Geometry check sheet. Reference: drawing and pictorial views, mm from the part's lowest x, y, z. A direction names the side the tool comes from. Coordinates: 2 decimals unless noted, no trailing zeros. Write each loop counter-clockwise with the first axis right and the second up, starting at its lowest first coordinate (ties: lowest second). Pieces come first, ordered by that corner, then holes.
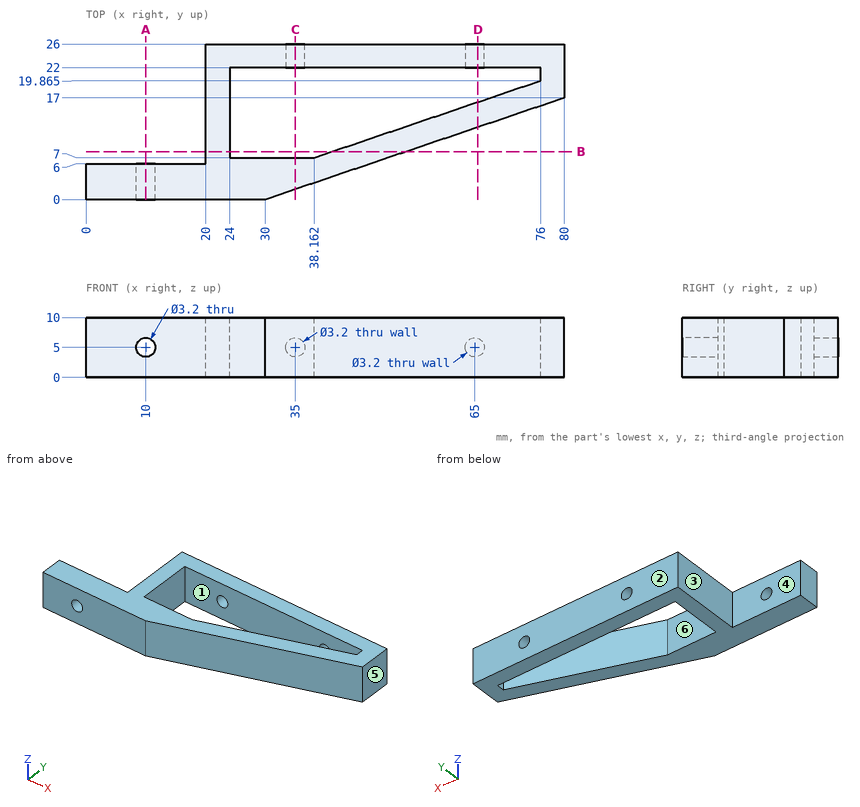
1. Sectioned sample at D-D, the plane x = 65.5. Record the boundary of the cut face in (y, z) (3 decimals), and give its area (3 significant figures).
2. Gauge pin test, flat ends, axial feed: P1, Ø4, axis at x = 65, z = 5, coming from the -Y side; P2, Ø6, axis at y = 23, z = 2.5, coming from the -X side. Record the tip position at first contact, or that the pin passes through.
3. Tool access check on the marked faces 1, 2 and 3. Record the directions out of +Z, -Z, +X, -X, +Y, -Y that give a thin tool (end or side, any length) a straight path to the whole face; none if there is none.
4. Sectioned sample at A-A, the plane x = 10. Record the boundary of the cut face in (y, z).
5. Sectioned sample at C-C, the plane x = 35. Record the boundary of the cut face in (y, z), and give its area (3 significant figures).
6. Draft check along Y on the marked faces 4, 5 and 6. Enter one of: pulls with the +Y half, pulls with the -Y half, needs draft (parallel to the pull), parting line crosses it, or undercut.
7. Sectioned sample at B-B, the plane y = 8. Record the boundary of the cut face in (x, z), and give its area (3 significant figures).
8. Material ranges on L1, parallel to Z at x = 65, y = 24.6; L2, parallel to X at y = 22.25, z = 7; L3, parallel to Y at x = 7, z = 2.5, recorded low to high.
Outcome:
1. outline: (12.07, 0) - (16.295, 0) - (16.295, 10) - (12.07, 10) - close; (22, 0) - (26, 0) - (26, 3.48) - (22, 3.48) - close; (22, 6.52) - (26, 6.52) - (26, 10) - (22, 10) - close
1. area: 70.1 mm2
2. P1: stops at y = 11.22
2. P2: stops at x = 20
3. face 1: +Z, -Z
3. face 2: +Z, -Z, +X, -X, +Y
3. face 3: +Z, -Z, -X, +Y
4. outline: (0, 0) - (6, 0) - (6, 3.4) - (0, 3.4) - close; (0, 6.6) - (6, 6.6) - (6, 10) - (0, 10) - close
5. outline: (1.7, 0) - (7, 0) - (7, 10) - (1.7, 10) - close; (22, 0) - (26, 0) - (26, 3.4) - (22, 3.4) - close; (22, 6.6) - (26, 6.6) - (26, 10) - (22, 10) - close
5. area: 80.2 mm2
6. face 4: pulls with the +Y half
6. face 5: needs draft
6. face 6: undercut
7. outline: (20, 0) - (24, 0) - (24, 10) - (20, 10) - close; (41.1, 0) - (53.53, 0) - (53.53, 10) - (41.1, 10) - close
7. area: 164 mm2
8. L1: z = 0 to 3.4, 6.6 to 10
8. L2: x = 20 to 80
8. L3: y = 0 to 6
